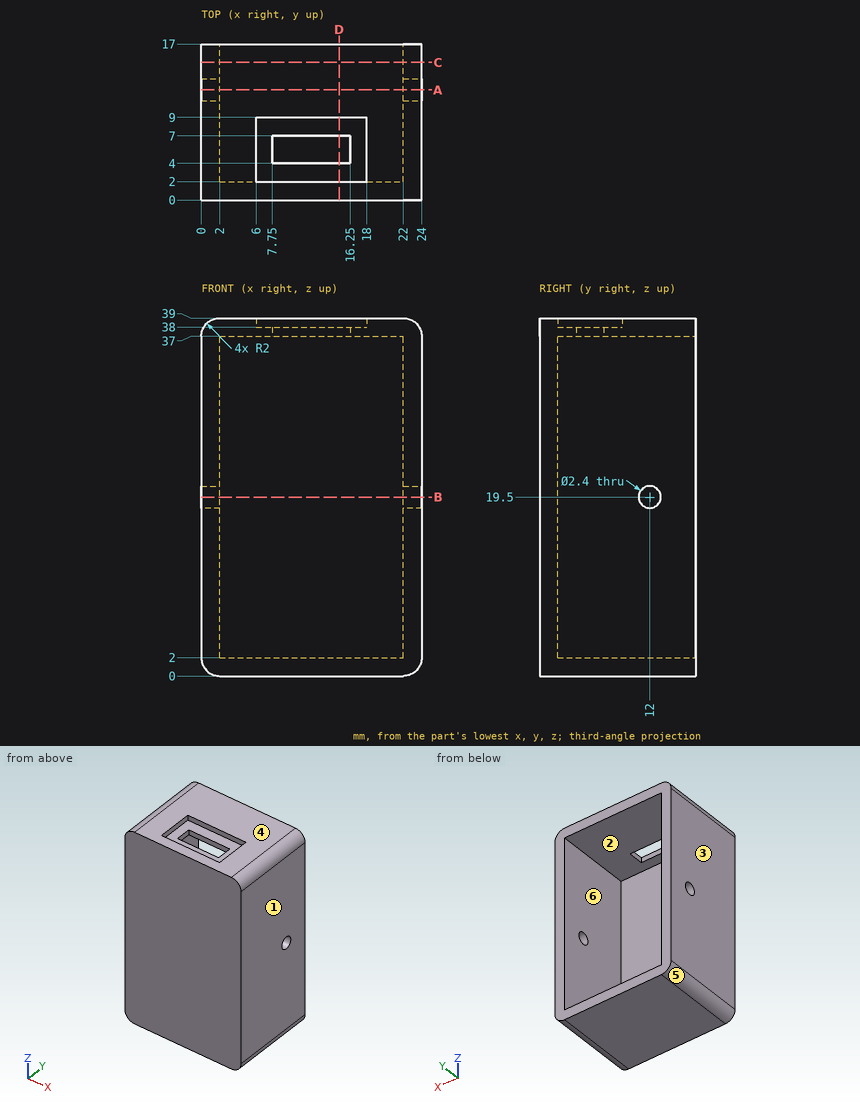
Verification items for this drawing (mm, ordinates from the low corner). A direction names the side the tool comes from. Round coordinates to 2 decimals unless told otherwise and drop trailing zeros. Write each loop counter-clockwise with the first axis right and the second up, starting at its lowest first coordinate (ties: lowest second). Pieces come first, ordered by that corner, then holes. Notation, with made-up numbers: M -6,61 L 27,61 A22 cw 27,76 Z; hole C 89,-11 d6. An arc over 180 degrees is marked long. Write item = value, one per line. Start each with the question number.
1. Scan lines: line 1 (Y direction, x = 0.75, z = 19.5); line 2 (X direction, y = 6.5, z = 10); line 3 (Z direction, x = 7.25, y = 16). Record each from-to range of solid material in increasing order. Write a range as [from, to].
2. Section check C-C, the plane y = 15. Record the cut outline in (x, z).
3. Release check for a two-part mould opening along Z. For the marked faces 3, 4, 5 and 6 record: pulls with the +Z half, pulls with the -Z half, needs draft (parallel to the pull), parting line crosses it, or undercut.
4. Section check D-D, the plane x = 15. Record the cut outline in (y, z), then the cut area to 3 significant figures.
5. Gauge pin test, flat ends, axial feed: pin 1 (0.8 mm diameter, centred on y = 6.5, z = 38.5, fed in from -X); pin 2 (4 mm diameter, centred on x = 11.5, z = 10.5, fed in from +Y); pin 3 (1.4 mm diameter, centred on y = 12, z = 19.5, fed in from -X) (1 decimal). Record the tip position at first contact, or that the pin passes through.
6. Section check B-B, the plane z = 19.5. Record the cut outline in (x, y).
7. Tool access check on the marked faces 1 and 2. Record the directions out of +Z, -Z, +X, -X, +Y, -Y that give a thin tool (end or side, any length) a straight path to the whole face; none if there is none.
8. Section check A-A, the plane y = 12. Record the cut outline in (x, z), then the cut area to 3 significant figures.
Results found:
q1.line_1 = [0, 10.8], [13.2, 17]
q1.line_2 = [0, 2], [22, 24]
q1.line_3 = [0, 2], [37, 39]
q2.outline = M 0,2 A2 ccw 2,0 L 22,0 A2 ccw 24,2 L 24,37 A2 ccw 22,39 L 2,39 A2 ccw 0,37 Z; hole M 2,2 L 22,2 L 22,37 L 2,37 Z
q3.face_3 = needs draft
q3.face_4 = pulls with the +Z half
q3.face_5 = pulls with the -Z half
q3.face_6 = undercut
q4.outline = M 0,0 L 17,0 L 17,2 L 2,2 L 2,37 L 4,37 L 4,38 L 2,38 L 2,39 L 0,39 Z; M 7,37 L 17,37 L 17,39 L 9,39 L 9,38 L 7,38 Z
q4.area = 128 mm^2
q5.pin_1 = 0.33
q5.pin_2 = 2
q5.pin_3 = through
q6.outline = M 0,0 L 24,0 L 24,10.8 L 22,10.8 L 22,2 L 2,2 L 2,10.8 L 0,10.8 Z; M 0,13.2 L 2,13.2 L 2,17 L 0,17 Z; M 22,13.2 L 24,13.2 L 24,17 L 22,17 Z
q7.face_1 = +Z, -Z, +X, +Y, -Y
q7.face_2 = +Y
q8.outline = M 0,2 A2 ccw 2,0 L 22,0 A2 ccw 24,2 L 24,18.3 L 22,18.3 L 22,2 L 2,2 L 2,18.3 L 0,18.3 Z; M 0,20.7 L 2,20.7 L 2,37 L 22,37 L 22,20.7 L 24,20.7 L 24,37 A2 ccw 22,39 L 2,39 A2 ccw 0,37 Z
q8.area = 223 mm^2
